Here's how the part is built. I have some questions about the finished solid (model axes, mm). A direction names the side the tool comes from. Round coordinates to 2 decimals unless told otherwise and drop trailing zeros. Loops run counter-clockwise (first coordinate to the right, second up) from the corner with the lowest first, then second, coordinate; pieces in that order, holes last. Notation, with made-up numbers: (-9.5, -9.5) -> (6.5, -9.5) arc R17 ccw to (6.5, 3.5) -> close; hole circle Ø1 at (15, 0). An arc over 180 degrees is marked (long way). Use one line per item in the form item = value. Start each with the question number.
Item 1: If we section it at A-A (x = -46): Write out the boundary of the cut face in (y, z).
Item 2: Thinking about a two-plate mould opening in X: for faces 4 (the face through (1, 39.947, 2)), 5 (the face through (64.691, 32, 2)), 6 (the face through (-25.309, -38, 2)), which applies, released by +X, released by -X, zero draft, split by the parting line, or undercut?
Item 3: For faces 1 (the face through (67, 7.398, 2)), 2 (the face through (24.691, -38, 2)), 3 (the face through (42, -20.079, 2)), which set-ups out of +Z, -Z, +X, -X, +Y, -Y let a thin tool reach every point of the face, with its end or its side?
Item 4: I'm going to push flat-ended pins straight in: pin 1 Ø3 at (y, z) = (-6, 3) entering from -X; pin 2 Ø2.5 at (y, z) = (-38.5, 3) entering from +X; pin 3 Ø2.5 at (x, z) = (-2, 2) entering from -Y. Where does each tip first touch, or does it pass through?
Item 5: If I drill on L1, parallel to Y at x = -44.5, z = 0.7; L2, parallel to X at y = 28.5, z = 1.8; L3, parallel to X at y = -35.5, z = 1.4, over which ranges is the centre line in solid material (lowest first)? Write a range as [from, to].
Item 6: If we section it at D-D (y = 32): Write out the boundary of the cut face in (x, z).
Item 7: If we section it at C-C (y = -3): Write out the boundary of the cut face in (x, z).
Item 8: If we section it at B-B (z = 3.2): State how many separate pieces and enclosed holes the cut face has, then the cut area to 3 significant figures.
```python
from build123d import *

# Parameters (mm, degrees)
SKETCH1_W           = 10
SKETCH1_H           = 5
SKETCH1_W_2         = 15
SKETCH1_W_3         = 14.993943351
BOSS_EXTRUDE2_DEPTH = 5


with BuildPart() as part:
    # Sketch1 → Boss-Extrude2 (new body)
    with BuildSketch(Plane.XY):
        Polygon((64.690886285, 24.89766958), (64.690886285, 39.946939566), (-65.309113715, 39.946939566), (-65.309113715, 24.89766958), (-70.309113715, 24.89766958), (-70.309113715, 7.39766958), (-65.309113715, 7.39766958), (-65.309113715, -7.60233042), (-70.309113715, -7.60233042), (-70.309113715, -25.10233042), (-65.309113715, -25.10233042), (-65.309113715, -40.053060434), (-50.309113715, -40.079299927), (-50.309113715, -35.079299927), (-35.309113715, -35.079299927), (-35.309113715, -40.079299927), (-25.309113715, -40.079299927), (-25.309113715, -35.079299927), (-15.309113715, -35.079299927), (-15.309113715, -40.079299927), (-5.309113715, -40.079299927), (-5.309113715, -35.079299927), (4.690886285, -35.079299927), (4.690886285, -40.079299927), (14.690886285, -40.079299927), (14.690886285, -35.079299927), (24.690886285, -35.079299927), (24.690886285, -40.079299927), (34.690886285, -40.079299927), (34.690886285, -35.079299927), (49.684829636, -35.079299927), (49.684829636, -40.079299927), (64.684829636, -40.079299927), (64.565827504, -25.10233042), (69.565827504, -25.10233042), (69.565827504, -7.60233042), (64.565827504, -7.60233042), (64.565827504, 7.39766958), (69.565827504, 7.39766958), (69.565827504, 24.89766958), align=None)
        with Locations((-0.309113715, -17.579299927)):
            Rectangle(SKETCH1_W, SKETCH1_H, mode=Mode.SUBTRACT)
        with Locations((-20.309113715, -17.579299927)):
            Rectangle(SKETCH1_W, SKETCH1_H, mode=Mode.SUBTRACT)
        with Locations((-42.809113715, -17.579299927)):
            Rectangle(SKETCH1_W_2, SKETCH1_H, mode=Mode.SUBTRACT)
        with Locations((42.187857961, -17.579299927)):
            Rectangle(SKETCH1_W_3, SKETCH1_H, mode=Mode.SUBTRACT)
        with Locations((19.690886285, -17.579299927)):
            Rectangle(SKETCH1_W, SKETCH1_H, mode=Mode.SUBTRACT)
    extrude(amount=BOSS_EXTRUDE2_DEPTH)


solid = part.part
```
Values found:
q1.outline = (-35.08, 0) -> (-20.08, 0) -> (-20.08, 5) -> (-35.08, 5) -> close; (-15.08, 0) -> (39.95, 0) -> (39.95, 5) -> (-15.08, 5) -> close
q2.face_4 = zero draft
q2.face_5 = released by +X
q2.face_6 = undercut
q3.face_1 = +Z, -Z, +X
q3.face_2 = +Z, -Z, -Y
q3.face_3 = +Z, -Z
q4.pin_1 = -65.31
q4.pin_2 = 64.68
q4.pin_3 = -35.08
q5.L1 = [-35.08, -20.08], [-15.08, 39.95]
q5.L2 = [-65.31, 64.69]
q5.L3 = [-65.31, -50.31], [-35.31, -25.31], [-15.31, -5.31], [4.69, 14.69], [24.69, 34.69], [49.68, 64.65]
q6.outline = (-65.31, 0) -> (64.69, 0) -> (64.69, 5) -> (-65.31, 5) -> close
q7.outline = (-65.31, 0) -> (64.57, 0) -> (64.57, 5) -> (-65.31, 5) -> close
q8.separate_pieces = 1
q8.enclosed_holes = 5
q8.area = 10,100 mm2
